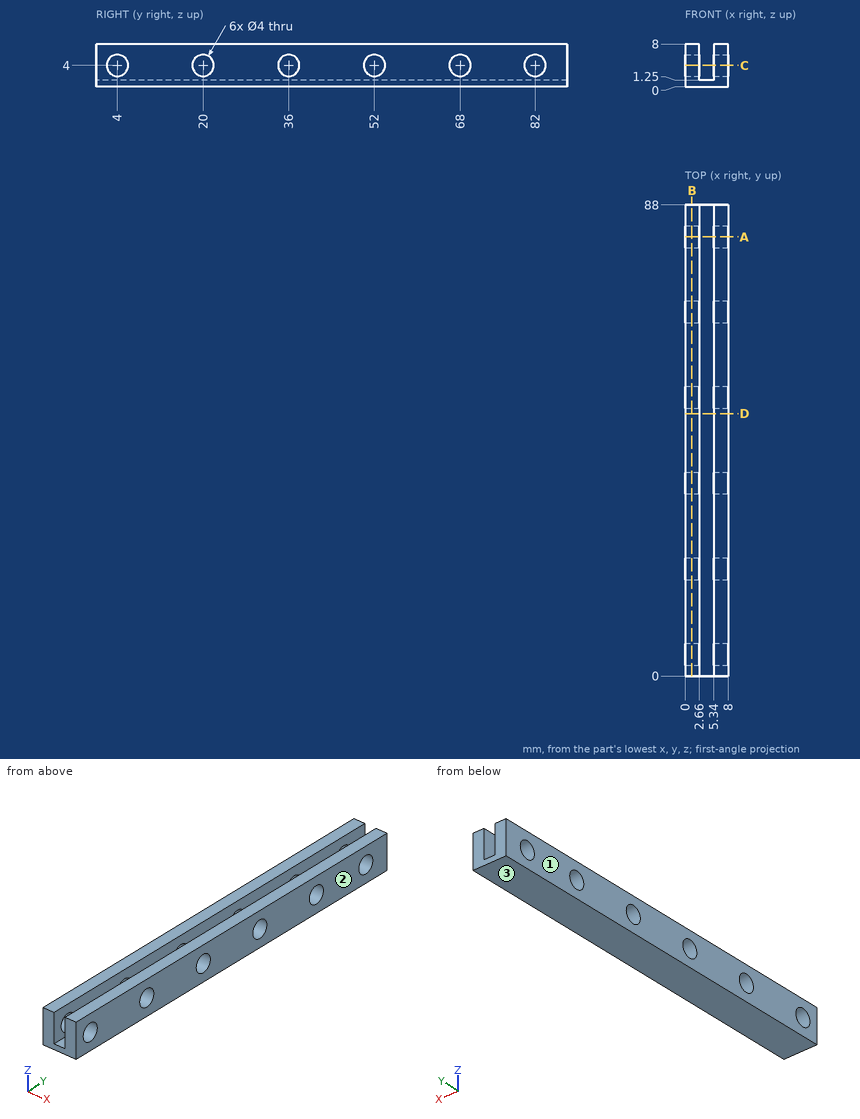
Geometry check sheet. Reference: drawing and pictorial views, mm from the part's lowest x, y, z. Give positions to 0.01 mm unless a question says otherwise; leave off trailing zeros. Order: outer loops, then holes, each group sorted by start corner. A loop starts at its lowest first (then second) coordinate and runs counter-clockwise, first axis right, second up. Notation, with made-up numbers: M -3,12.25 L 37,12.25 A14 cw 37,17.25 Z; hole C 89,38.25 d10. An arc over 180 degrees is marked long. Return JSON: item names as keys, results as strings. Group by question number.
1) Mould release check, pull along X, two halves, no side actions. Record for the marked faces 1, 2 and 3: pulls with the +X half, pulls with the -X half, needs draft (parallel to the pull), parting line crosses it, or undercut.
2) Section check B-B on x = 1.25. Record the cut outline in (y, z).
3) Go/stop test with a flat-tipped pin: pin 1 Ø1 at (x, y) = (4.5, 28.5) entering from +Z. Record where the tip stops, or that it passes through.
4) Section check C-C on z = 4. Give the number of separate pieces and of enclosed holes in the cut face, and give its area (3 significant figures).
5) Scan lines: line 1 (Z direction, x = 6.5, y = 52); line 2 (X direction, y = 54, z = 3.5); line 3 (Z direction, x = 3.75, y = 24.5). Record each from-to range of solid material in increasing order.
6) Section check A-A on y = 82. Record the cut outline in (x, z), and give its area (3 significant figures).
7) Section check D-D on y = 49. Record the cut outline in (x, z), and give its area (3 significant figures).
Answer block:
{
 "1": {"face 1": "pulls with the -X half", "face 2": "pulls with the +X half", "face 3": "needs draft"},
 "2": {"outline": "M 0,0 L 88,0 L 88,8 L 0,8 Z; hole C 4,4 d4; hole C 20,4 d4; hole C 36,4 d4; hole C 52,4 d4; hole C 68,4 d4; hole C 82,4 d4"},
 "3": {"pin 1": "stops at z = 1.25"},
 "4": {"separate pieces": "14", "enclosed holes": "0", "area": "340 mm^2"},
 "5": {"line 1": "z = 0 to 2, 6 to 8", "line 2": "x = 0 to 2.66, 5.34 to 8", "line 3": "z = 0 to 1.25"},
 "6": {"outline": "M 0,0 L 8,0 L 8,2 L 5.34,2 L 5.34,1.25 L 2.66,1.25 L 2.66,2 L 0,2 Z; M 0,6 L 2.66,6 L 2.66,8 L 0,8 Z; M 5.34,6 L 8,6 L 8,8 L 5.34,8 Z", "area": "24.6 mm^2"},
 "7": {"outline": "M 0,0 L 8,0 L 8,8 L 5.34,8 L 5.34,1.25 L 2.66,1.25 L 2.66,8 L 0,8 Z", "area": "45.9 mm^2"}
}
